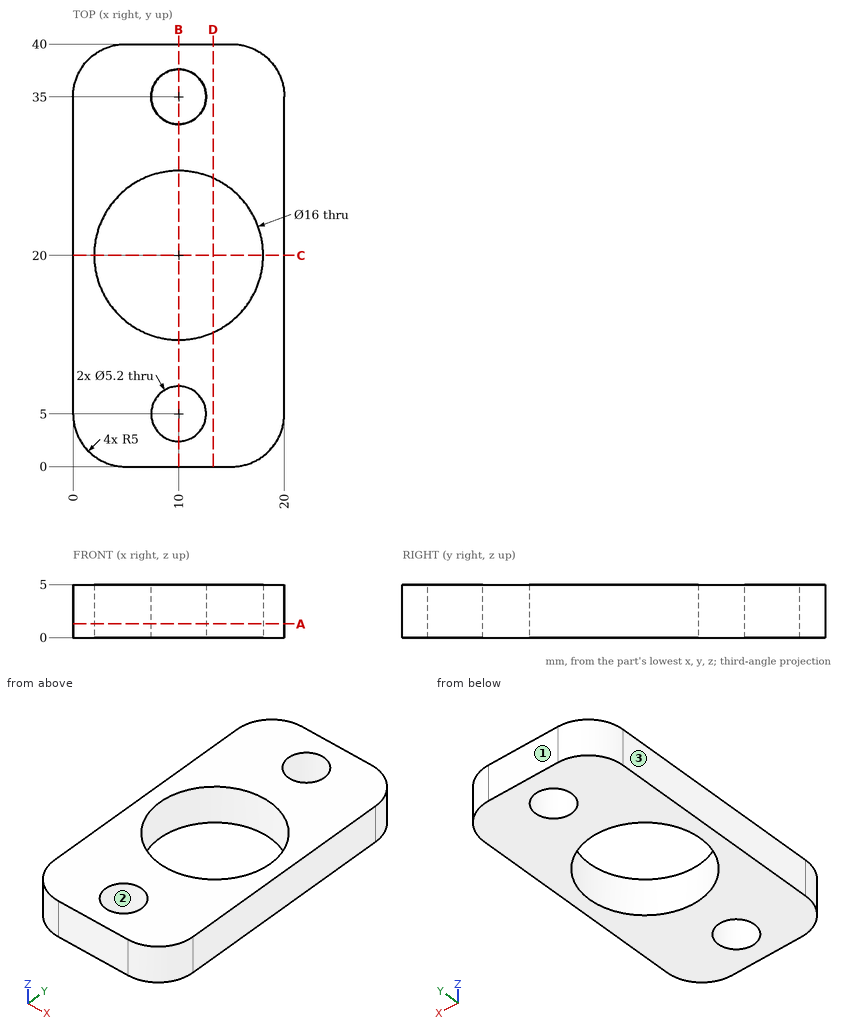
Geometry check sheet. Reference: drawing and pictorial views, mm from the part's lowest x, y, z. Give positions to 0.01 mm unless a question says otherwise; leave off trailing zeros. Order: outer loops, then holes, each group sorted by start corner. A loop starts at its lowest first (then second) coordinate and runs counter-clockwise, first axis right, second up. Notation, with made-up numbers: (81, 1.5) -> (128, 1.5) arc R27 cw to (128, 21.5) -> close; hole circle Ø7 at (24, -10.5). An arc over 180 degrees is marked (long way). Write each question's results on one line, items separated by ' | '. Start each with the question number.
(1) Gauge pin test, flat ends, axial feed: P1, Ø3, axis at x = 10.5, z = 2, coming from the -Y side; P2, Ø3, axis at x = 10, y = 5, coming from the -Z side. Record the tip position at first contact, or that the pin passes through.
(2) Sectioned sample at D-D (x = 13.25). Enter the section's corners in (y, z), plus the area to 3 significant figures.
(3) Mould release check, pull along X, two halves, no side actions. Record for the marked faces 1, 2 and 3: pulls with the +X half, pulls with the -X half, needs draft (parallel to the pull), parting line crosses it, or undercut.
(4) Scan lines: line 1 (Y direction, x = 10, z = 3.9); line 2 (Y direction, x = 8.25, z = 3.3); line 3 (X direction, y = 35, z = 1.75). Record each from-to range of solid material in increasing order.
(5) Sectioned sample at C-C (y = 20). Enter the section's corners in (x, z).
(6) Sectioned sample at B-B (x = 10). Enter the section's corners in (y, z).
(7) Sectioned sample at A-A (z = 1.3). Enter the section's corners in (x, y), plus the area to 3 significant figures.
Answer below:
1) P1: y = 0 | P2: through
2) outline: (0, 0) -> (12.69, 0) -> (12.69, 5) -> (0, 5) -> close; (27.31, 0) -> (40, 0) -> (40, 5) -> (27.31, 5) -> close | area: 127 mm2
3) face 1: needs draft | face 2: undercut | face 3: pulls with the -X half
4) line 1: 0 to 2.4, 7.6 to 12, 28 to 32.4, 37.6 to 40 | line 2: 0 to 3.08, 6.92 to 12.19, 27.81 to 33.08, 36.92 to 40 | line 3: 0 to 7.4, 12.6 to 20
5) outline: (0, 0) -> (2, 0) -> (2, 5) -> (0, 5) -> close; (18, 0) -> (20, 0) -> (20, 5) -> (18, 5) -> close
6) outline: (0, 0) -> (2.4, 0) -> (2.4, 5) -> (0, 5) -> close; (7.6, 0) -> (12, 0) -> (12, 5) -> (7.6, 5) -> close; (28, 0) -> (32.4, 0) -> (32.4, 5) -> (28, 5) -> close; (37.6, 0) -> (40, 0) -> (40, 5) -> (37.6, 5) -> close
7) outline: (0, 5) arc R5 ccw to (5, 0) -> (15, 0) arc R5 ccw to (20, 5) -> (20, 35) arc R5 ccw to (15, 40) -> (5, 40) arc R5 ccw to (0, 35) -> close; hole circle Ø16 at (10, 20); hole circle Ø5.2 at (10, 5); hole circle Ø5.2 at (10, 35) | area: 535 mm2
